Drawing for the job (mm, zero at the part's lowest x, y, z). A direction names the side the tool comes from. Give positions to 0.01 mm unless a question says otherwise; leave off trailing zeros. Loops run counter-clockwise (first coordinate to the right, second up) from the corner with the lowest first, then second, coordinate; pieces in that order, holes last. Notation, with made-up numbers: (45.5, 63) -> (59.5, 63) arc R27 ccw to (59.5, 96) -> close; hole circle Ø3 at (77.5, 24.5). An arc over 180 degrees is marked (long way). Use CSV: the item, a comma, the result in double quotes. Start each with the question number.
(1) Cut at A-A on y = 12.5. Write the cut outline in (x, z), then the cut area to 3 significant figures.
(2) Cut at C-C on z = 13.5. Write the cut outline in (x, y).
(3) Flat gauge pins, fed straight in: pin 1 (1 mm diameter, centred on x = 10, z = 13.5, fed in from -Y); pin 2 (2 mm diameter, centred on x = 3.5, y = 14.5, fed in from +Z); pin 3 (10 mm diameter, centred on y = 20, z = 18, fed in from -X); pin 4 (11.5 mm diameter, centred on x = 15, y = 18, fed in from +Z). Where does each tip first touch, or does it go through?
(4) 3-axis set-ups, long thin cutter, end or side, ignore diameter. For the marked faces 1 and 2: which of +Z, -Z, +X, -X, +Y, -Y reach the whole face in a straight line?
(5) Drill centre lines: probe 1 along Z at (x, y) = (11.75, 22.75); probe 2 along Z at (x, y) = (18, 10.75); probe 3 along Y at (x, z) = (11, 16.25). Where is each one in solid material? Low to high.
(6) Cut at B-B on z = 2. Write the cut outline in (x, y), then the cut area to 3 significant figures.
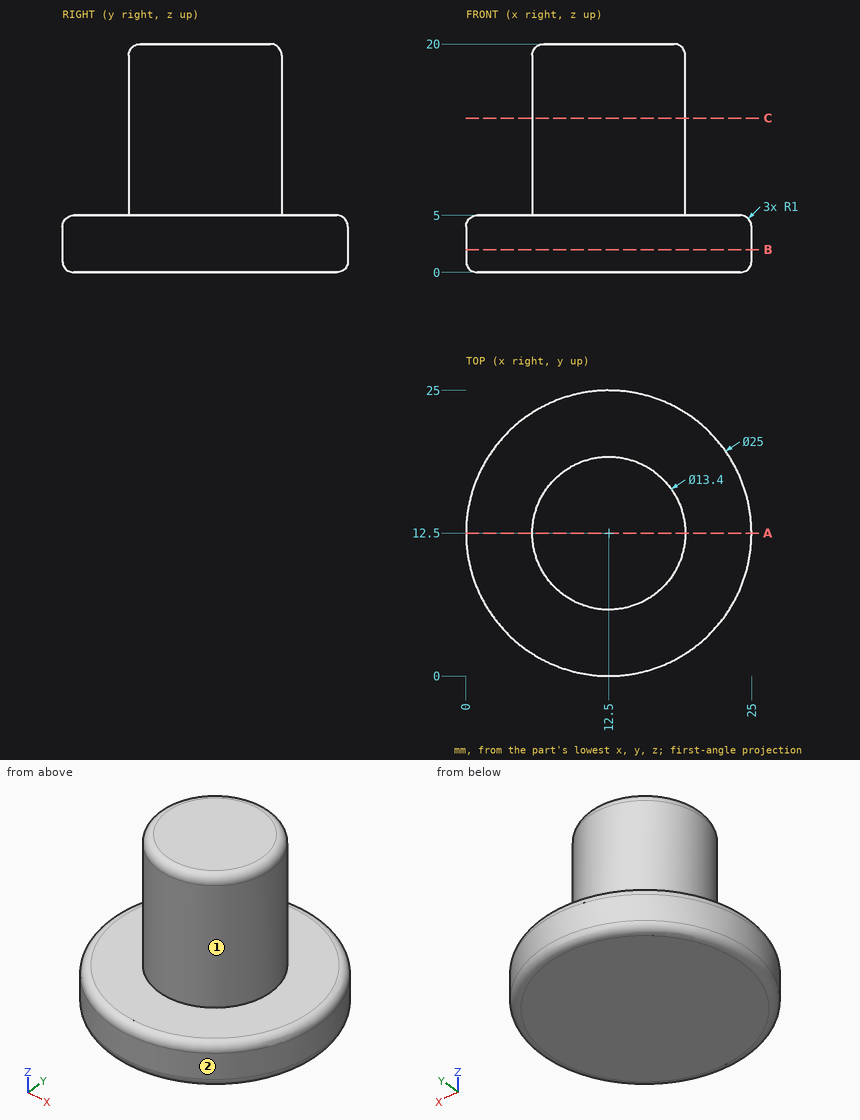
Check result:
1,outline,"(0, 1) arc R1 ccw to (1, 0) -> (24, 0) arc R1 ccw to (25, 1) -> (25, 4) arc R1 ccw to (24, 5) -> (19.2, 5) -> (19.2, 19) arc R1 ccw to (18.2, 20) -> (6.8, 20) arc R1 ccw to (5.8, 19) -> (5.8, 5) -> (1, 5) arc R1 ccw to (0, 4) -> close"
1,area,"325 mm²"
2,outline,"circle Ø13.4 at (12.5, 12.5)"
3,pin 1,"y = 6.11"
3,pin 2,"z = 5"
3,pin 3,"x = 6.28"
3,pin 4,"z = 20"
4,face 1,"+Z"
4,face 2,"+Z, -Z"
5,probe 1,"0 to 5"
5,probe 2,"0 to 20"
5,probe 3,"5.97 to 19.03"
6,outline,"circle Ø25 at (12.5, 12.5)"
6,area,"491 mm²"
